from build123d import *

# Parameters (mm, degrees)
SKETCH1_R           = 2.38125
BOSS_EXTRUDE1_DEPTH = 3.175


with BuildPart() as part:
    # Sketch1 → Boss-Extrude1 (new body)
    with BuildSketch(Plane(origin=(0, 0, 0), x_dir=(1, 0, 0), z_dir=(0, 1, 0))):
        with BuildLine():
            Line((-10.16, -38.1), (6.35, -38.1))
            Line((6.35, -38.1), (60.96, -38.1))
            ThreePointArc((60.96, -38.1), (62.756051224, -37.356051224), (63.5, -35.56))
            Line((63.5, -35.56), (63.5, -15.24))
            ThreePointArc((63.5, -15.24), (62.756051224, -13.443948776), (60.96, -12.7))
            Line((60.96, -12.7), (19.05, -12.7))
            ThreePointArc((19.05, -12.7), (14.559871939, -10.840128061), (12.7, -6.35))
            Line((12.7, -6.35), (12.7, 35.56))
            ThreePointArc((12.7, 35.56), (11.956051224, 37.356051224), (10.16, 38.1))
            Line((10.16, 38.1), (-10.16, 38.1))
            ThreePointArc((-10.16, 38.1), (-11.956051224, 37.356051224), (-12.7, 35.56))
            Line((-12.7, 35.56), (-12.7, -35.56))
            ThreePointArc((-12.7, -35.56), (-11.956051224, -37.356051224), (-10.16, -38.1))
        make_face()
        with Locations(Location((0, -25.4, 0), (0, 0, 270))):
            Circle(SKETCH1_R, mode=Mode.SUBTRACT)
        with Locations(Location((0, 0, 0), (0, 0, 270))):
            Circle(SKETCH1_R, mode=Mode.SUBTRACT)
        with Locations(Location((0, 25.4, 0), (0, 0, 270))):
            Circle(SKETCH1_R, mode=Mode.SUBTRACT)
        with Locations(Location((25.4, -25.4, 0), (0, 0, 270))):
            Circle(SKETCH1_R, mode=Mode.SUBTRACT)
        with Locations(Location((50.8, -25.4, 0), (0, 0, 270))):
            Circle(SKETCH1_R, mode=Mode.SUBTRACT)
    extrude(amount=BOSS_EXTRUDE1_DEPTH)


solid = part.part
Design review of the part built by this model. Coordinates are the model's own, in mm. A direction names the side the tool comes from. Coordinates: 2 decimals unless noted, no trailing zeros. Write each loop counter-clockwise with the first axis right and the second up, starting at its lowest first coordinate (ties: lowest second). Pieces come first, ordered by that corner, then holes. Notation, with made-up numbers: (62.5, 69) - (94.5, 69) arc R13 cw to (94.5, 77) - close; hole circle Ø7 at (83, 51). An arc over 180 degrees is marked (long way). Use one line per item in the form item = value.
Q1. Consider section C-C (y = 1.95). Write out the cut boundary in (x, z), plus the area to 3 significant figures.
Taken from the geometry:
outline = (-12.7, -35.56) arc R2.54 ccw to (-10.16, -38.1) - (10.16, -38.1) arc R2.54 ccw to (12.7, -35.56) - (12.7, 6.35) arc R6.35 cw to (19.05, 12.7) - (60.96, 12.7) arc R2.54 ccw to (63.5, 15.24) - (63.5, 35.56) arc R2.54 ccw to (60.96, 38.1) - (-10.16, 38.1) arc R2.54 ccw to (-12.7, 35.56) - close; hole circle Ø4.76 at (0, -25.4); hole circle Ø4.76 at (0, 0); hole circle Ø4.76 at (0, 25.4); hole circle Ø4.76 at (25.4, 25.4); hole circle Ø4.76 at (50.8, 25.4)
area = 3,140 mm^2
Q2. The part is to be moulded in two halves that separate along Z. For faces 1 (the cylindrical face through (-1.45, 1.57, -1.89)), 2 (the cylindrical face through (-11.976, 1.565, 37.336)), 3 (the cylindrical face through (14.61, 1.57, 10.89)), 4 (the cylindrical face through (25.5, 1.57, 23.02)), say which applies: +Z half, -Z half, draft (parallel to the pull), parting line (faces both ways), or undercut.
Taken from the geometry:
face_1 = undercut
face_2 = +Z half
face_3 = -Z half
face_4 = undercut
Q3. Consider section A-A (x = 0). Write out the cut boundary in (y, z) (3 decimals).
Taken from the geometry:
outline = (0, -38.1) - (3.175, -38.1) - (3.175, -27.781) - (0, -27.781) - close; (0, -23.019) - (3.175, -23.019) - (3.175, -2.381) - (0, -2.381) - close; (0, 2.381) - (3.175, 2.381) - (3.175, 23.019) - (0, 23.019) - close; (0, 27.781) - (3.175, 27.781) - (3.175, 38.1) - (0, 38.1) - close
Q4. Insertion check: pin 1 Ø4.5 at (x, z) = (50.8, 25.4) entering from -Y. The pin has a flat end and moves straight along its axis. Give the tip position at first contact, or say it passes through.
Taken from the geometry:
pin_1 = through
Q5. Machinability: for faces 5 (the flat face through (40, 2, 12.7)), 6 (the flat face through (8, 3.175, 8)), which of the approach directions +Z, -Z, +X, -X, +Y, -Y give a long, thin tool a straight path to every point of the face, cutting with its end or side? Answer none if there is none.
Taken from the geometry:
face_5 = -Z, +X, +Y, -Y
face_6 = +Z, -Z, +X, -X, +Y
Q6. Consider section B-B (z = 25.4). Write out the cut boundary in (x, y) (3 decimals).
Taken from the geometry:
outline = (-12.7, 0) - (-2.381, 0) - (-2.381, 3.175) - (-12.7, 3.175) - close; (2.381, 0) - (23.019, 0) - (23.019, 3.175) - (2.381, 3.175) - close; (27.781, 0) - (48.419, 0) - (48.419, 3.175) - (27.781, 3.175) - close; (53.181, 0) - (63.5, 0) - (63.5, 3.175) - (53.181, 3.175) - close
Q7. For probe 1 along X at (y, z) = (1.7, 25.4); probe 2 along Z at (x, y) = (-1.5, 3); probe 3 along X at (y, z) = (1.05, 0), list the stretches that pass through material, from the lowest coordinate up.
Taken from the geometry:
probe_1 = -12.7 to -2.38, 2.38 to 23.02, 27.78 to 48.42, 53.18 to 63.5
probe_2 = -38.1 to -27.25, -23.55 to -1.85, 1.85 to 23.55, 27.25 to 38.1
probe_3 = -12.7 to -2.38, 2.38 to 12.7
Q8. Consider section D-D (z = -25.4). Write out the cut boundary in (x, y) (3 decimals), plus the area to 3 significant figures.
Taken from the geometry:
outline = (-12.7, 0) - (-2.381, 0) - (-2.381, 3.175) - (-12.7, 3.175) - close; (2.381, 0) - (12.7, 0) - (12.7, 3.175) - (2.381, 3.175) - close
area = 65.5 mm^2
